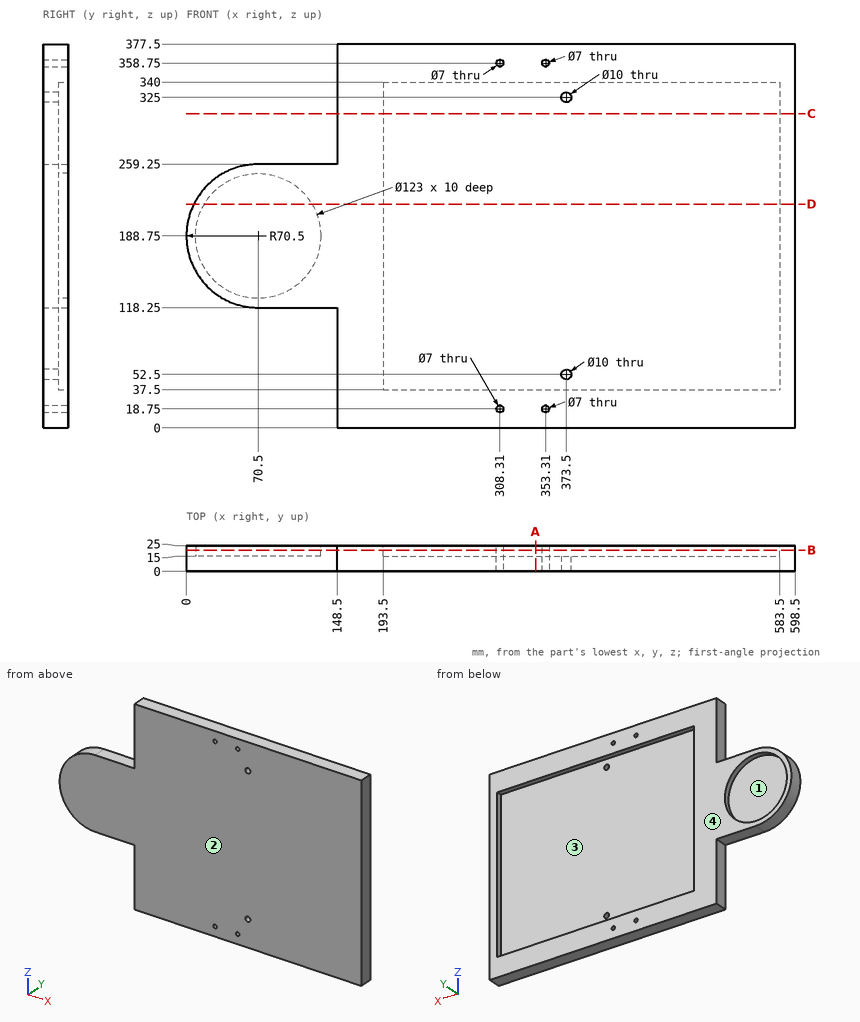
Source: three-view drawing plus pictorial views. Frame: mm from the lowest corner of the part. A direction names the side the tool comes from. Round coordinates to 2 decimals unless told otherwise and drop trailing zeros. Loops run counter-clockwise (first coordinate to the right, second up) from the corner with the lowest first, then second, coordinate; pieces in that order, holes last. Notation, with made-up numbers: M -20,-36.5 L 19,-36.5 A21 ccw 19,-29.5 Z; hole C 50.25,68.5 d4. An arc over 180 degrees is marked long. Answer as CSV lines item,"result".
Q1. Line query: line 1 along X through (y, z) = (17.25, 188.75); line 2 along Z through (x, y) = (373.5, 3.5); line 3 along X through (y, z) = (22, 359). Output: solid intervals per line, ascending.
Verdict:
line 1,"x = 0 to 9, 132 to 193.5, 583.5 to 598.5"
line 2,"z = 0 to 47.5, 57.5 to 320, 330 to 377.5"
line 3,"x = 148.5 to 304.82, 311.8 to 349.82, 356.8 to 598.5"
Q2. Reachability of the marked faces 1 and 2 from +Z, -Z, +X, -X, +Y, -Y: full face, straight path, thin tool, end or side. Return the list, or none.
Verdict:
face 1,"+Y"
face 2,"+Z, -Z, +X, -X, -Y"
Q3. Pull-direction query (Z, two-part tool) for the marked faces 3 and 4; classes: +Z half, -Z half, draft (parallel to the pull), parting line (faces both ways), or undercut.
Verdict:
face 3,"undercut"
face 4,"draft"
Q4. Cut plane A-A (x = 343.5). Return the cut outline in (y, z).
Verdict:
outline,"M 0,0 L 25,0 L 25,37.5 L 15,37.5 L 15,340 L 25,340 L 25,377.5 L 0,377.5 Z"
Q5. Cut plane B-B (y = 20.75). Return the cut outline in (x, z), plus the area to 3 significant figures.
Verdict:
outline,"M 70.5,118.25 L 148.5,118.25 L 148.5,0 L 598.5,0 L 598.5,377.5 L 148.5,377.5 L 148.5,259.25 L 70.5,259.25 A70.5 ccw Z; hole C 70.5,188.75 d123; hole M 193.5,37.5 L 583.5,37.5 L 583.5,340 L 193.5,340 Z; hole C 308.31,18.75 d7; hole C 308.31,358.75 d7; hole C 353.31,18.75 d7; hole C 353.31,358.75 d7"
area,"58,700 mm^2"
Q6. Contact query for flat-ended pins moving along their axis: pin 1 (5.5 mm diameter, centred on x = 353.31, z = 358.75, fed in from -Y); pin 2 (11.5 mm diameter, centred on x = 373.5, z = 52.5, fed in from +Y); pin 3 (12.5 mm diameter, centred on x = 125.5, y = 15, fed in from +Z); pin 4 (7.5 mm diameter, centred on y = 14, z = 85, fed in from -X). Output: stop coordinate, or through.
Verdict:
pin 1,"passes through"
pin 2,"stops at y = 15"
pin 3,"stops at z = 259.25"
pin 4,"stops at x = 148.5"
Q7. Cut plane D-D (z = 220). Return the cut outline in (x, y).
Verdict:
outline,"M 7.3,0 L 598.5,0 L 598.5,25 L 583.5,25 L 583.5,15 L 193.5,15 L 193.5,25 L 123.47,25 L 123.47,15 L 17.53,15 L 17.53,25 L 7.3,25 Z"
Q8. Cut plane C-C (z = 309). Return the cut outline in (x, y).
Verdict:
outline,"M 148.5,0 L 598.5,0 L 598.5,25 L 583.5,25 L 583.5,15 L 193.5,15 L 193.5,25 L 148.5,25 Z"
